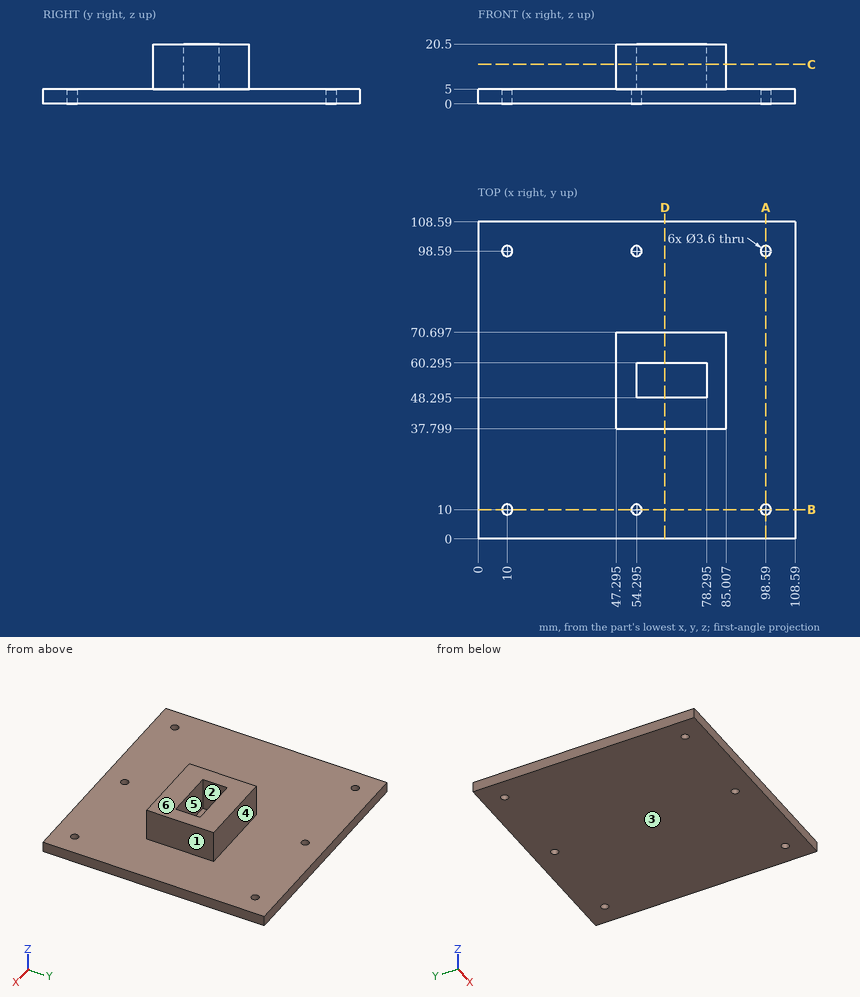
Answer from the drawing. Dimensions are ordinates in mm from the lowest x, y and z of the part. A direction names the side the tool comes from. Give positions to 0.01 mm unless a question says otherwise; leave off trailing zeros. Order: outer loops, then holes, each group sorted by start corner. A loop starts at its lowest first (then second) coordinate and runs counter-clockwise, first axis right, second up.
(1) Given pin 1 (4.5 mm diameter, centred on x = 98.59, y = 10, fed in from +Z); pin 2 (8 mm diameter, centred on y = 50, z = 16.5, fed in from -X) (3 decimals); pin 3 (2 mm diameter, centred on x = 54.295, y = 98.59, fed in from -Z); pin 4 (4.5 mm diameter, centred on x = 74, z = 10.5, fed in from +Y), each flat-ended and moving along its own axis, determine where each tip first touches the part or whether it passes through.
(2) For a pull along X with two mould halves and no side action, classify the marked faces 1, 2 and 3 as released by +X, released by -X, zero draft, split by the parting line, or undercut.
(3) Find section B-B (y = 10). Give the vertices of the cut face in (x, z) (1 decimal).
(4) Find section A-A (x = 98.59). Give the vertices of the cut face in (y, z), plus the area to 3 significant figures.
(5) Find section D-D (x = 64). Give the vertices of the cut face in (y, z) (1 decimal), plus the area to 3 significant figures.
(6) Straight lines are drawn through the part: L1, parallel to Y at x = 98.59, z = 2.6; L2, parallel to X at y = 98.59, z = 1.1 (1 decimal); L3, parallel to Y at x = 58, z = 13.5 (1 decimal). For each, find the intervals that lie inside material, in ascending order.
(7) Find section C-C (z = 13.5). Give the vertices of the cut face in (x, y) (1 decimal).
(8) For the marked faces 4, 5 and 6, determine the directions among +Z, -Z, +X, -X, +Y, -Y from which every point of the face is accessible in a straight line to the end or side of a thin tool.
Result sheet:
1. pin 1: stops at z = 5
1. pin 2: stops at x = 47.295
1. pin 3: passes through
1. pin 4: stops at y = 70.7
2. face 1: released by +X
2. face 2: undercut
2. face 3: zero draft
3. outline: (0, 0) - (8.2, 0) - (8.2, 5) - (0, 5) - close; (11.8, 0) - (52.5, 0) - (52.5, 5) - (11.8, 5) - close; (56.1, 0) - (96.8, 0) - (96.8, 5) - (56.1, 5) - close; (100.4, 0) - (108.6, 0) - (108.6, 5) - (100.4, 5) - close
4. outline: (0, 0) - (8.2, 0) - (8.2, 5) - (0, 5) - close; (11.8, 0) - (96.79, 0) - (96.79, 5) - (11.8, 5) - close; (100.39, 0) - (108.59, 0) - (108.59, 5) - (100.39, 5) - close
4. area: 507 mm2
5. outline: (0, 0) - (108.6, 0) - (108.6, 5) - (70.7, 5) - (70.7, 20.5) - (60.3, 20.5) - (60.3, 5) - (48.3, 5) - (48.3, 20.5) - (37.8, 20.5) - (37.8, 5) - (0, 5) - close
5. area: 867 mm2
6. L1: y = 0 to 8.2, 11.8 to 96.79, 100.39 to 108.59
6. L2: x = 0 to 8.2, 11.8 to 52.5, 56.1 to 96.8, 100.4 to 108.6
6. L3: y = 37.8 to 48.3, 60.3 to 70.7
7. outline: (47.3, 37.8) - (85, 37.8) - (85, 70.7) - (47.3, 70.7) - close; hole (54.3, 48.3) - (78.3, 48.3) - (78.3, 60.3) - (54.3, 60.3) - close
8. face 4: +Z, +X, -X, +Y
8. face 5: +Z
8. face 6: +Z, +X, -X, +Y, -Y
